Check sheet for the modelled part. Datum: model origin and axes. Units: mm. Face numbers are marked on the shaded views. A direction names the side the tool comes from. Coordinates: 2 decimals unless noted, no trailing zeros. Loops run counter-clockwise (first coordinate to the right, second up) from the corner with the lowest first, then second, coordinate; pieces in that order, holes last. Notation, with made-up numbers: (-26.75, -36.5) - (15.25, -36.5) arc R29 ccw to (15.25, -7.5) - close; hole circle Ø9 at (-22, -14.75). An arc over 180 degrees is marked (long way). Use a Markdown table: item, result. Add a question column.
1) Tool access check on the marked faces 1, 2 and 3. Record the directions out of +Z, -Z, +X, -X, +Y, -Y that give a thin tool (end or side, any length) a straight path to the whole face; none if there is none.
2) Thickness scan on line 1 (Z direction, x = -1.5, y = 0.75); line 2 (X direction, y = -0.1, z = 3.5); line 3 (X direction, y = 0, z = -0.5). Record the ranges inside material, lowest first.
3) Sectioned sample at D-D, the plane y = 1.65. Enter the section's corners in (x, z), then the cut area to 3 significant figures.
4) Sectioned sample at A-A, the plane y = 0. Enter the section's corners in (x, z) (3 decimals).
5) Go/stop test with a flat-tipped pin: P1, Ø1, axis at y = -1, z = 1.5, coming from the -X side. Record where the tip stops, or that it passes through.
6) Sectioned sample at C-C, the plane z = 5. Enter the section's corners in (x, y), then the cut area to 3 significant figures.
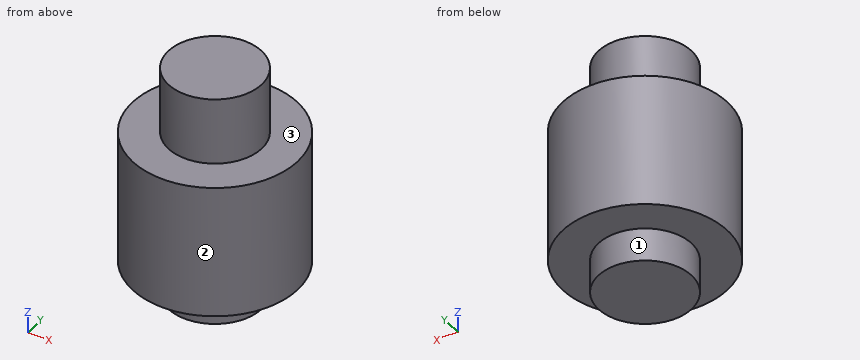
from build123d import *

# Parameters (mm, degrees)
F0_R     = 2.475
F0_R_2   = 1.5
F1_DEPTH = 4
F2_R     = 1.4
F3_DEPTH = 2
F4_R     = 1.4
F5_DEPTH = 1


with BuildPart() as f1:
    # F0 (on Top) → F1 (new body)
    with BuildSketch(Plane.XY):
        Circle(F0_R)
        Circle(F0_R_2, mode=Mode.SUBTRACT)
        Circle(F0_R_2)
    extrude(amount=F1_DEPTH)

    # F2 (on face) → F3 (join)
    with BuildSketch(Plane.XY.offset(4)):
        Circle(F2_R)
    extrude(amount=F3_DEPTH)

    # F4 (on face) → F5 (join)
    with BuildSketch(Plane(origin=(0, 0, 0), x_dir=(1, 0, 0), z_dir=(0, 0, -1))):
        Circle(F4_R)
    extrude(amount=F5_DEPTH)


solid = f1.part
Solved:
| question | item | result |
|---|---|---|
| 1 | face 1 | -Z |
| 1 | face 2 | +Z, -Z |
| 1 | face 3 | +Z |
| 2 | line 1 | z = 0 to 4 |
| 2 | line 2 | x = -2.47 to 2.47 |
| 2 | line 3 | x = -1.4 to 1.4 |
| 3 | outline | (-1.84, 0) - (1.84, 0) - (1.84, 4) - (-1.84, 4) - close |
| 3 | area | 14.8 mm2 |
| 4 | outline | (-2.475, 0) - (-1.4, 0) - (-1.4, -1) - (1.4, -1) - (1.4, 0) - (2.475, 0) - (2.475, 4) - (1.4, 4) - (1.4, 6) - (-1.4, 6) - (-1.4, 4) - (-2.475, 4) - close |
| 5 | P1 | stops at x = -2.42 |
| 6 | outline | circle Ø2.8 at (0, 0) |
| 6 | area | 6.16 mm2 |
